from build123d import *

# Parameters (mm, degrees)
SKETCH1_R           = 28.448
EXTRUDE1_DEPTH      = 82.55
CUT_EXTRUDE1_DEPTH  = 34.1376
SKETCH13_W          = 11.3284
SKETCH13_H          = 19.05
S2D0011_W           = 5.4991
S2D0011_H           = 16.002
SKETCH16_W          = 76.2
SKETCH16_H          = 25.4
EXTRUDE2_DEPTH      = 31.75
EXTRUDE2_DEPTH_BACK = 31.75
SKETCH17_R          = 10.4775
CUT_EXTRUDE9_DEPTH  = 0.254
SKETCH18_R          = 10.4775
CUT_EXTRUDE10_DEPTH = 0.254
CIRPATTERN2_COUNT   = 6
HOLE1_D             = 7.1374
HOLE1_DEPTH         = 25.4
CUT_EXTRUDE11_DEPTH = 4.0386
CUT_EXTRUDE12_DEPTH = 3.175


with BuildPart() as part:
    # Sketch1 → Extrude1 (new body)
    with BuildSketch(Plane.XY):
        Circle(SKETCH1_R)
    extrude(amount=EXTRUDE1_DEPTH)

    # Sketch2 → Cut-Extrude1 (cut, symmetric)
    with BuildSketch(Plane(origin=(0, 0, 0), x_dir=(0, 0, 1), z_dir=(1, 0, 0))):
        with BuildLine():
            Line((69.342, 28.448), (69.342, 25.781))
            ThreePointArc((69.342, 25.781), (69.490789755, 25.421789755), (69.85, 25.273))
            Line((69.85, 25.273), (82.55, 25.273))
            Line((82.55, 25.273), (82.55, 28.448))
            Line((82.55, 28.448), (69.342, 28.448))
        make_face()
    cut_extrude1 = extrude(amount=CUT_EXTRUDE1_DEPTH, both=True, mode=Mode.SUBTRACT)

    # Sketch10 → Cut-Revolve1 (revolve, cut)
    with BuildSketch(Plane(origin=(0, 0, 0), x_dir=(0, 0, -1), z_dir=(1, 0, 0)), mode=Mode.PRIVATE) as cut_revolve1_sk:
        Polygon((-82.55, 27.432), (-69.85, 27.432), (-68.834, 28.448), (-82.55, 28.448), align=None)
    revolve(cut_revolve1_sk.sketch.rotate(Axis((0, 0, 83.2358), (0, 0, -1)), 90), axis=Axis((0, 0, 83.2358), (0, 0, -1)), mode=Mode.SUBTRACT)  # turned: the seam where the file's is

    # Sketch13 → Revolve1 (revolve)
    with BuildSketch(Plane(origin=(0, 0, 0), x_dir=(0, 0, -1), z_dir=(1, 0, 0)), mode=Mode.PRIVATE) as revolve1_sk:
        with Locations((-88.2142, 9.525)):
            Rectangle(SKETCH13_W, SKETCH13_H)
    revolve(revolve1_sk.sketch.rotate(Axis((0, 0, 94.44482), (0, 0, -1)), 90), axis=Axis((0, 0, 94.44482), (0, 0, -1)))  # turned: the seam where the file's is

    # S2D0011 → Cut-Revolve4 (revolve, cut)
    with BuildSketch(Plane(origin=(-5.4991, 0, 93.8784), x_dir=(-1, 0, 0), z_dir=(0, 1, 0)), mode=Mode.PRIVATE) as cut_revolve4_sk:
        with Locations((-2.74955, -8.001)):
            Rectangle(S2D0011_W, S2D0011_H)
    revolve(cut_revolve4_sk.sketch.rotate(Axis((0, 0, 39.576937479), (0, 0, 1)), 180), axis=Axis((0, 0, 39.576937479), (0, 0, 1)), mode=Mode.SUBTRACT)  # turned: the seam where the file's is

    # Sketch15 → Cut-Revolve5 (revolve, cut)
    with BuildSketch(Plane(origin=(0, 0, 0), x_dir=(0, 0, -1), z_dir=(1, 0, 0)), mode=Mode.PRIVATE) as cut_revolve5_sk:
        with BuildLine():
            Line((-93.8784, 14.2875), (-89.706615474, 18.79729325))
            ThreePointArc((-89.706615474, 18.79729325), (-89.444021381, 18.984062482), (-89.1286, 19.05))
            Line((-89.1286, 19.05), (-93.8784, 19.05))
            Line((-93.8784, 19.05), (-93.8784, 14.2875))
        make_face()
    revolve(cut_revolve5_sk.sketch.rotate(Axis((0, 0, 94.11589), (0, 0, -1)), 90), axis=Axis((0, 0, 94.11589), (0, 0, -1)), mode=Mode.SUBTRACT)  # turned: the seam where the file's is

    # Sketch16 → Extrude2 (add, two sides)
    with BuildSketch(Plane(origin=(0, 0, 0), x_dir=(-1, 0, 0), z_dir=(0, 1, 0))) as extrude2_sk:
        with Locations((-6.35, 1.524)):
            Rectangle(SKETCH16_W, SKETCH16_H)
    extrude(amount=EXTRUDE2_DEPTH)
    extrude(extrude2_sk.sketch, amount=-EXTRUDE2_DEPTH_BACK)

    # Sketch17 → Cut-Extrude9 (cut)
    with BuildSketch(Plane(origin=(44.45, 0, 0), x_dir=(0, 0, -1), z_dir=(1, 0, 0))):
        with Locations((1.651, -15.875)):
            Circle(SKETCH17_R)
    extrude(amount=-CUT_EXTRUDE9_DEPTH, mode=Mode.SUBTRACT)

    # Sketch18 → Cut-Extrude10 (cut)
    with BuildSketch(Plane(origin=(44.45, 0, 0), x_dir=(0, 0, -1), z_dir=(1, 0, 0))):
        with Locations((1.651, 15.875)):
            Circle(SKETCH18_R)
    extrude(amount=-CUT_EXTRUDE10_DEPTH, mode=Mode.SUBTRACT)

    # S2D0002 → Cut-Revolve6 (revolve, cut)
    with BuildSketch(Plane(origin=(44.196, -15.875, -1.651), x_dir=(0, -1, 0), z_dir=(0, 0, 1)), mode=Mode.PRIVATE) as cut_revolve6_sk:
        Polygon((0, 0), (6.1849, 0), (5.642306865, -2.5527), (4.9784, -3.216606865), (4.9784, -17.272), (0, -17.272), align=None)
    revolve(cut_revolve6_sk.sketch.rotate(Axis((26.0604, -15.875, -1.651), (1, 0, 0)), 270), axis=Axis((26.0604, -15.875, -1.651), (1, 0, 0)), mode=Mode.SUBTRACT)  # turned: the seam where the file's is

    # S2D0001 → Cut-Revolve7 (revolve, cut)
    with BuildSketch(Plane(origin=(44.196, 15.875, -1.651), x_dir=(0, -1, 0), z_dir=(0, 0, 1)), mode=Mode.PRIVATE) as cut_revolve7_sk:
        Polygon((0, 0), (6.1849, 0), (5.642306865, -2.5527), (4.9784, -3.216606865), (4.9784, -17.272), (0, -17.272), align=None)
    revolve(cut_revolve7_sk.sketch.rotate(Axis((26.0604, 15.875, -1.651), (1, 0, 0)), 270), axis=Axis((26.0604, 15.875, -1.651), (1, 0, 0)), mode=Mode.SUBTRACT)  # turned: the seam where the file's is

    # CirPattern2: Cut-Extrude1 ×6 about axis
    cirpattern2_axis = Axis((0, 0, 0), (0, 0, 1))
    for i in range(1, CIRPATTERN2_COUNT):
        add(cut_extrude1.rotate(cirpattern2_axis, i * 360 / CIRPATTERN2_COUNT), mode=Mode.SUBTRACT)

    # Hole1
    with Locations(Plane.XY.offset(14.224)):
        with Locations((-26.1874, -26.1874), (34.925, 0), (-26.1874, 26.1874)):
            Hole(HOLE1_D / 2, depth=HOLE1_DEPTH)

    # Sketch23 → Cut-Extrude11 (cut)
    with BuildSketch(Plane.XY.offset(93.8784)):
        with BuildLine():
            Line((-14.2875, 12.600390619), (-14.2875, -12.600390619))
            ThreePointArc((-14.2875, -12.600390619), (-19.05, 0), (-14.2875, 12.600390619))
        make_face()
        with BuildLine():
            Line((14.2875, 12.600390619), (14.2875, -12.600390619))
            ThreePointArc((14.2875, -12.600390619), (19.05, 0), (14.2875, 12.600390619))
        make_face()
    extrude(amount=-CUT_EXTRUDE11_DEPTH, mode=Mode.SUBTRACT)

    # Sketch25 → Cut-Revolve8 (revolve, cut)
    with BuildSketch(Plane(origin=(0, 0, 0), x_dir=(0, 0, -1), z_dir=(1, 0, 0)), mode=Mode.PRIVATE) as cut_revolve8_sk:
        Polygon((-93.8784, 8.5344), (-93.0656, 9.3472), (-93.8784, 10.16), align=None)
    revolve(cut_revolve8_sk.sketch.rotate(Axis((0, 0, 93.13164), (0, 0, -1)), 90), axis=Axis((0, 0, 93.13164), (0, 0, -1)), mode=Mode.SUBTRACT)  # turned: the seam where the file's is

    # Sketch26 → Cut-Extrude12 (cut)
    with BuildSketch(Plane.XY.offset(93.8784)):
        with BuildLine():
            Line((-1.5875, 9.211405517), (-1.5875, -9.211405517))
            ThreePointArc((-1.5875, -9.211405517), (0, -9.3472), (1.5875, -9.211405517))
            Line((1.5875, -9.211405517), (1.5875, 9.211405517))
            ThreePointArc((1.5875, 9.211405517), (0, 9.3472), (-1.5875, 9.211405517))
        make_face()
    extrude(amount=-CUT_EXTRUDE12_DEPTH, mode=Mode.SUBTRACT)


solid = part.part
Build history of the part. All positions in model axes, mm. A direction names the side the tool comes from. Coordinates: 2 decimals unless noted, no trailing zeros. Write each loop counter-clockwise with the first axis right and the second up, starting at its lowest first coordinate (ties: lowest second). Pieces come first, ordered by that corner, then holes.
(1) Drill centre lines: line 1 (Z direction, x = 5, y = -29); line 2 (Z direction, x = 1, y = -26); line 3 (Z direction, x = 34.5, y = -11.5). Where is each one in solid material? Low to high.
(2) Cut at A-A on z = 72.5. List the corners of the cut face in (x, y), and give its area (3 significant figures).
(3) Pin check, flat tips, straight feed: pin 1 Ø1 at (y, z) = (9, 38.5) entering from +X; pin 2 Ø19 at (x, y) = (19.5, -14.5) entering from +Z; pin 3 Ø1 at (y, z) = (-6.5, 92) entering from +X. Stop position of each tip, or through.
(4) 3-axis set-ups, long thin cutter, end or side, ignore diameter. For faces 4 (the cylindrical face through (-27.43, -0.05, 76.11)), 5 (the flat face through (0, 7, 90.703)), 6 (the cylindrical face through (33.853, 20.735, -2.73)): which of +Z, -Z, +X, -X, +Y, -Y reach the whole face in a straight line?
(5) Mould opens along X. For faces 1 (the cylindrical face through (-13.675, -23.781, 76.111)), 2 (the flat face through (-1.588, -7, 92)), 3 (the flat face through (-23, 13, 69.342)) say: pulls with the +X half, pulls with the -X half, needs draft (parallel to the pull), parting line crosses it, or undercut.
(6) Cut at C-C on x = -26. State how many separate pieces and enclosed holes the cut face has, and give its area (3 significant figures).
Working result:
1. line 1: z = -11.18 to 14.22
1. line 2: z = -11.18 to 69.34
1. line 3: z = -11.18 to -4.03, 0.72 to 14.22
2. outline: (-27.22, -3.4) - (-16.55, -21.87) arc R27.43 ccw to (-10.67, -25.27) - (10.67, -25.27) arc R27.43 ccw to (16.55, -21.87) - (27.22, -3.4) arc R27.43 ccw to (27.22, 3.4) - (16.55, 21.87) arc R27.43 ccw to (10.67, 25.27) - (-10.67, 25.27) arc R27.43 ccw to (-16.55, 21.87) - (-27.22, 3.4) arc R27.43 ccw to start
2. area: 2,180 mm2
3. pin 1: stops at x = 27.15
3. pin 2: stops at z = 93.4
3. pin 3: stops at x = 14.29
4. face 4: +Z, -X
4. face 5: +Z
4. face 6: +X
5. face 1: pulls with the -X half
5. face 2: undercut
5. face 3: needs draft
6. separate pieces: 3
6. enclosed holes: 0
6. area: 2,670 mm2
